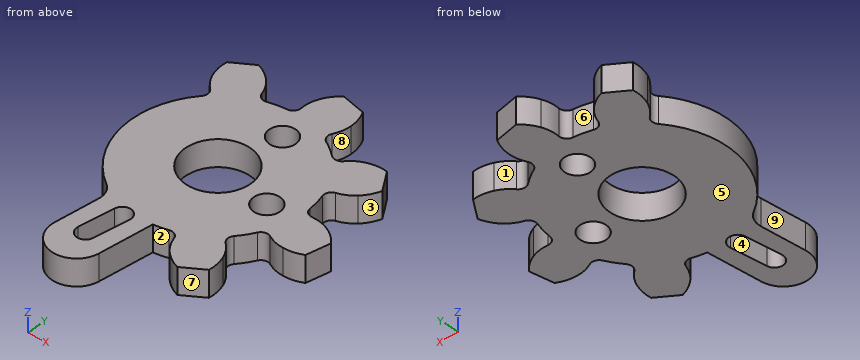
```python
from build123d import *

# Parameters (mm, degrees)
SKETCH1_R           = 1.5
SKETCH1_R_2         = 3.7
BOSS_EXTRUDE1_DEPTH = 3


with BuildPart() as part:
    # Sketch1 → Boss-Extrude1 (new body)
    with BuildSketch(Plane.XY):
        with BuildLine():
            Line((13.740457451, -4.042470891), (14.255332257, -1.392017357))
            ThreePointArc((14.255332257, -1.392017357), (13.480746798, -0.642737861), (12.546028185, -0.106357853))
            ThreePointArc((12.546028185, -0.106357853), (11.607127827, 0.157211053), (10.632288023, 0.1834752))
            ThreePointArc((10.632288023, 0.1834752), (10.010207796, 0.372487454), (9.703996042, 0.94602368))
            ThreePointArc((9.703996042, 0.94602368), (9.553721125, 1.946512948), (9.300578942, 2.926043632))
            ThreePointArc((9.300578942, 2.926043632), (9.357660457, 3.573428685), (9.855662757, 3.990992351))
            ThreePointArc((9.855662757, 3.990992351), (10.742650685, 4.396276035), (11.503786091, 5.005927856))
            ThreePointArc((11.503786091, 5.005927856), (12.154418131, 5.865043883), (12.57442922, 6.85751206))
            Line((12.57442922, 6.85751206), (11.06434702, 9.095737194))
            ThreePointArc((11.06434702, 9.095737194), (9.986811776, 9.077843176), (8.946587965, 8.796175247))
            ThreePointArc((8.946587965, 8.796175247), (8.096313795, 8.318643798), (7.388426402, 7.647899519))
            ThreePointArc((7.388426402, 7.647899519), (6.814897409, 7.341674219), (6.192821647, 7.530701165))
            ThreePointArc((6.192821647, 7.530701165), (5.379108488, 8.131893498), (4.507477145, 8.645527732))
            ThreePointArc((4.507477145, 8.645527732), (4.09006951, 9.14366082), (4.146948213, 9.791063724))
            ThreePointArc((4.146948213, 9.791063724), (4.487564551, 10.704837744), (4.594679622, 11.674130687))
            ThreePointArc((4.594679622, 11.674130687), (4.447259181, 12.741683783), (4.042470891, 13.740457451))
            Line((4.042470891, 13.740457451), (1.392017357, 14.255332257))
            ThreePointArc((1.392017357, 14.255332257), (0.642737861, 13.480746798), (0.106357853, 12.546028185))
            ThreePointArc((0.106357853, 12.546028185), (-0.157211053, 11.607127827), (-0.1834752, 10.632288023))
            ThreePointArc((-0.1834752, 10.632288023), (-0.372487454, 10.010207796), (-0.94602368, 9.703996042))
            ThreePointArc((-0.94602368, 9.703996042), (-1.946512948, 9.553721125), (-2.926043632, 9.300578942))
            ThreePointArc((-2.926043632, 9.300578942), (-3.573428685, 9.357660457), (-3.990992351, 9.855662757))
            ThreePointArc((-3.990992351, 9.855662757), (-4.396276035, 10.742650685), (-5.005927856, 11.503786091))
            ThreePointArc((-5.005927856, 11.503786091), (-5.865043883, 12.154418131), (-6.85751206, 12.57442922))
            Line((-6.85751206, 12.57442922), (-9.095737194, 11.06434702))
            ThreePointArc((-9.095737194, 11.06434702), (-9.077843176, 9.986811776), (-8.796175247, 8.946587965))
            ThreePointArc((-8.796175247, 8.946587965), (-8.318643798, 8.096313795), (-7.647899519, 7.388426402))
            ThreePointArc((-7.647899519, 7.388426402), (-7.341674219, 6.814897409), (-7.530701165, 6.192821647))
            ThreePointArc((-7.530701165, 6.192821647), (-9.635448804, -1.490176611), (-5.308108038, -8.178416047))
            ThreePointArc((-5.308108038, -8.178416047), (-4.590564776, -8.998081228), (-4.409043882, -10.072217861))
            Line((-4.409043882, -10.072217861), (-4.952379844, -15.064191543))
            ThreePointArc((-4.952379844, -15.064191543), (-2.426769985, -18.205915305), (0.714311062, -15.679506151))
            Line((0.714311062, -15.679506151), (1.370494976, -9.653198615))
            ThreePointArc((1.370494976, -9.653198615), (2.155492092, -9.508751433), (2.926043632, -9.300578942))
            ThreePointArc((2.926043632, -9.300578942), (3.573428685, -9.357660457), (3.990992351, -9.855662757))
            ThreePointArc((3.990992351, -9.855662757), (4.396276035, -10.742650685), (5.005927856, -11.503786091))
            ThreePointArc((5.005927856, -11.503786091), (5.865043883, -12.154418131), (6.85751206, -12.57442922))
            Line((6.85751206, -12.57442922), (9.095737194, -11.06434702))
            ThreePointArc((9.095737194, -11.06434702), (9.077843176, -9.986811776), (8.796175247, -8.946587965))
            ThreePointArc((8.796175247, -8.946587965), (8.318643798, -8.096313795), (7.647899519, -7.388426402))
            ThreePointArc((7.647899519, -7.388426402), (7.341674219, -6.814897409), (7.530701165, -6.192821647))
            ThreePointArc((7.530701165, -6.192821647), (8.131893498, -5.379108488), (8.645527732, -4.507477145))
            ThreePointArc((8.645527732, -4.507477145), (9.14366082, -4.09006951), (9.791063724, -4.146948213))
            ThreePointArc((9.791063724, -4.146948213), (10.704837744, -4.487564551), (11.674130687, -4.594679622))
            ThreePointArc((11.674130687, -4.594679622), (12.741683783, -4.447259181), (13.740457451, -4.042470891))
        make_face()
        with Locations((6.625050503, -1.101923166)):
            Circle(SKETCH1_R, mode=Mode.SUBTRACT)
        with Locations((0.002221487, -0.000323095)):
            Circle(SKETCH1_R_2, mode=Mode.SUBTRACT)
        with Locations((1.303084957, 6.668993396)):
            Circle(SKETCH1_R, mode=Mode.SUBTRACT)
        with BuildLine():
            Line((-3.068510764, -14.155643998), (-2.492411625, -10.197347675))
            ThreePointArc((-2.492411625, -10.197347675), (-1.35881276, -9.351798379), (-0.513263464, -10.485397245))
            Line((-0.513263464, -10.485397245), (-1.089362603, -14.443693568))
            ThreePointArc((-1.089362603, -14.443693568), (-2.222961468, -15.289242864), (-3.068510764, -14.155643998))
        make_face(mode=Mode.SUBTRACT)
    extrude(amount=BOSS_EXTRUDE1_DEPTH)


solid = part.part
```
Verification items for the finished model (mm, model axes). Face numbers are marked on the shaded views. A direction names the side the tool comes from. Give positions to 0.01 mm unless a question says otherwise; leave off trailing zeros. Loops run counter-clockwise (first coordinate to the right, second up) from the corner with the lowest first, then second, coordinate; pieces in that order, holes last. Notation, with made-up numbers: M -26.5,-16.5 L 4.5,-16.5 A23 ccw 4.5,-7.5 Z; hole C 71,62.25 d3. An arc over 180 degrees is marked long. Return JSON: item names as keys, results as strings.
1) Section check C-C, the plane y = -5.5. Enter the section's corners in (x, z), and give its area (3 significant figures).
Findings:
{"outline": "M -8.05,0 L 8.05,0 L 8.05,3 L -8.05,3 Z", "area": "48.3 mm2"}
2) Material ranges on L1, parallel to X at y = -11, z = 2; L2, parallel to Y at x = 7.75, z = 1.2; L3, parallel to X at y = -10, z = 0.6, recorded low to high. Write a range as [from, to].
Findings:
{"L1": "x = [-4.51, -2.61], [-0.59, 1.22], [4.57, 9.1]", "L2": "y = [-11.97, -7.48], [-5.92, -2.09], [-0.11, 8.03]", "L3": "x = [-4.4, -2.44], [-0.56, 1.33], [4.04, 9.08]"}
3) Gauge pin test, flat ends, axial feed: P1, Ø6.5, axis at x = 0, y = 0, coming from the -Z side; P2, Ø1, axis at y = 9.5, z = 1.5, coming from the +X side. Record the tip position at first contact, or that the pin passes through.
Findings:
{"P1": "passes through", "P2": "stops at x = 11.13"}
4) Section check A-A, the plane y = 2.5. Enter the section's corners in (x, z).
Findings:
{"outline": "M -9.42,0 L -2.73,0 L -2.73,3 L -9.42,3 Z; M 2.73,0 L 9.42,0 L 9.42,3 L 2.73,3 Z"}
5) Mould release check, pull along Y, two halves, no side actions. Record for the marked faces 6, 7, 8 and 9: released by +Y, released by -Y, zero draft, split by the parting line, or undercut.
Findings:
{"face 6": "released by +Y", "face 7": "released by -Y", "face 8": "undercut", "face 9": "undercut"}
6) Section check B-B, the plane z = 0.9. Count the separate pieces of the cut face and the enclosed holes in it, and give its area (3 significant figures).
Findings:
{"separate pieces": "1", "enclosed holes": "4", "area": "376 mm2"}
7) Tool access check on the marked faces 1, 2, 3, 4 and 5. Record the directions out of +Z, -Z, +X, -X, +Y, -Y that give a thin tool (end or side, any length) a straight path to the whole face; none if there is none.
Findings:
{"face 1": "+Z, -Z, +Y", "face 2": "+Z, -Z, -Y", "face 3": "+Z, -Z, +X", "face 4": "+Z, -Z", "face 5": "-Z, +X, -X, +Y, -Y"}
